Build history of the part. All positions in model axes, mm. A direction names the side the tool comes from. Round coordinates to 2 decimals unless told otherwise and drop trailing zeros. Loops run counter-clockwise (first coordinate to the right, second up) from the corner with the lowest first, then second, coordinate; pieces in that order, holes last.
Autodesk Inventor part; units mm, degrees
ref_plane "YZ Plane" through (0, 0, 0) normal (1, 0, 0) x (0, 1, 0)
ref_plane "XZ Plane" through (0, 0, 0) normal (0, 1, 0) x (-1, 0, 0)
ref_plane "XY Plane" through (0, 0, 0) normal (0, 0, 1) x (1, 0, 0)
sketch "Sketch1" plane through (0, 0, 0) normal (0, 1, 0) x (-1, 0, 0)
  line L0 (20.25, -20.25) -> (-20.25, -20.25)
  line L1 (-20.25, -20.25) -> (-20.25, 20.25)
  line L2 (-20.25, 20.25) -> (20.25, 20.25)
  line L3 (20.25, 20.25) -> (20.25, -20.25)
  line L4 (23.25, 23.25) -> (-23.25, 23.25)
  line L5 (-23.25, 23.25) -> (-23.25, -23.25)
  line L6 (-23.25, -23.25) -> (23.25, -23.25)
  line L7 (23.25, -23.25) -> (23.25, 23.25)
  point P0 (0, 0)
  point P1 (20.25, 0)
  point P2 (0, -20.25)
  point P3 (23.25, 0)
  point P4 (0, -23.25)
  dimension "d0" = 40.5
  dimension "d1" = 40.5
  dimension "d2" = 46.5
  dimension "d3" = 46.5
extrude "Extrusion1" add sketch "Sketch1" along normal blind 10
fillet "Fillet1" radius 3 8 edges at (-23.25, 5, 23.25) (23.25, 5, 23.25) (23.25, 5, -23.25) (-23.25, 5, -23.25) (-20.25, 5, -20.25) (-20.25, 5, 20.25) (20.25, 5, 20.25) (20.25, 5, -20.25)
ref_plane "Arbeitsebene3" through (-17.25, 0, -20.25) normal (1, 0, 0) x (0, 1, 0)
sketch "Skizze10" plane through (0, 10, 0) normal (0, 1, 0) x (1, 0, 0)
  line L0 (20.25, 23.25) -> (-20.25, 23.25)
  arc A0 (-20.25, 23.25) -> (-23.25, 20.25) centre (-20.25, 20.25) ccw
  line L1 (-23.25, 20.25) -> (-23.25, -20.25)
  arc A1 (-23.25, -20.25) -> (-20.25, -23.25) centre (-20.25, -20.25) ccw
  line L2 (-20.25, -23.25) -> (20.25, -23.25)
  arc A2 (20.25, -23.25) -> (23.25, -20.25) centre (20.25, -20.25) ccw
  line L3 (23.25, -20.25) -> (23.25, 20.25)
  arc A3 (23.25, 20.25) -> (20.25, 23.25) centre (20.25, 20.25) ccw
  line L4 (-20.25, 23.25) -> (20.25, 23.25)
  line L5 (23.25, 20.25) -> (23.25, -20.25)
  line L6 (20.25, -23.25) -> (-20.25, -23.25)
  line L7 (-23.25, -20.25) -> (-23.25, 20.25)
  arc A4 (-20.25, 23.25) -> (-23.25, 20.25) centre (-20.25, 20.25) ccw
  arc A5 (23.25, 20.25) -> (20.25, 23.25) centre (20.25, 20.25) ccw
  arc A6 (20.25, -23.25) -> (23.25, -20.25) centre (20.25, -20.25) ccw
  arc A7 (-23.25, -20.25) -> (-20.25, -23.25) centre (-20.25, -20.25) ccw
  line L8 (-20.25, -23.25) -> (20.25, -23.25)
  point P0 (0, 0)
extrude "Extrusion6" add sketch "Skizze10" along normal blind 2
sketch "Skizze9" plane through (-17.25, 0, -20.25) normal (1, 0, 0) x (0, 1, 0)
  line L0 (12, 0) -> (0, 0) construction
  line L1 (6.2, 0) -> (6.2, 0.8787) construction
  line L2 (3.3, 0) -> (1.3, 0)
  line L3 (10, 3) -> (10, 37.5)
  line L4 (10, 20.25) -> (0, 20.25)
  line L5 (10, 40.5) -> (0, 40.5) construction
  ellipse E0 centre (2.3, 0) end of major axis (1.3, 0) minor radius 0.5
  line L6 (3.3, 0) -> (1.3, 0)
  line L7 (10, 40.5) -> (0, 40.5) construction
  line L8 (3.3, 40.5) -> (1.3, 40.5)
  ellipse E1 centre (2.3, 40.5) end of major axis (1.3, 40.5) minor radius 0.5
  point P0 (4.6, 0)
  point P1 (10, 0)
  point P2 (6.2, 3)
  point P3 (6.2, 15.294)
  point P4 (2.3, 0.5)
  dimension "d51" = 1.6
  dimension "d52" = 2.3
  dimension "d53" = 1
  dimension "d64" = 0.5
chamfer "Fasen1" distance 2 angle 45 8 edges at (-23.25, 12, 0) (-22.3713, 12, 22.3713) (0, 12, 23.25) (22.3713, 12, 22.3713) (23.25, 12, 0) (22.3713, 12, -22.3713) (0, 12, -23.25) (-22.3713, 12, -22.3713)
extrude "Extrusion7" add sketch "Skizze9" along normal blind 37.5 and the other way blind 5 contours L2 E0 | E1 L8 picked at (2.2882, 0.1666) picked at (2.3118, 40.3334)
properties part number "IMU_mount_cover"
(1) Probe line 1 (Z direction, x = -4, y = 8); line 2 (X direction, y = 8, z = -17.5); line 3 (Y direction, x = 8.5, z = -5). List the from-to ranges inside material, lowest first.
Responses:
line 1: z = -23.25 to -20.25, 20.25 to 23.25
line 2: x = -23.25 to -20.24, 20.24 to 23.25
line 3: y = 10 to 12
(2) Which spindle directions (+Z, -Z, +X, -X, +Y, -Y) get a long thin tool onto all of the face, cutting with end or side? Do faces 1 (the face through (0, 1, -20.25)), 2 (the face through (-22.35, 4.93, 22.39)), 3 (the face through (19.35, 5.07, 19.39)). Say none if no direction does.
Responses:
face 1: -Y
face 2: +Z, -X, +Y, -Y
face 3: none
(3) Slice it at B-B on z = -16. List the corners of the cut face in (x, y).
Responses:
outline: (-23.25, 0) - (-20.25, 0) - (-20.25, 10) - (20.25, 10) - (20.25, 0) - (23.25, 0) - (23.25, 10) - (21.25, 12) - (-21.25, 12) - (-23.25, 10) - close
(4) Slice it at A-A on y = 6.75. List the corners of the cut face in (x, z).
Responses:
outline: (-23.25, -20.25) arc R3 ccw to (-20.25, -23.25) - (20.25, -23.25) arc R3 ccw to (23.25, -20.25) - (23.25, 20.25) arc R3 ccw to (20.25, 23.25) - (-20.25, 23.25) arc R3 ccw to (-23.25, 20.25) - close; hole (-20.25, -17.25) arc R3 ccw to (-17.25, -20.25) - (17.25, -20.25) arc R3 ccw to (20.25, -17.25) - (20.25, 17.25) arc R3 ccw to (17.25, 20.25) - (-17.25, 20.25) arc R3 ccw to (-20.25, 17.25) - close
(5) Pull direction X, two halves, no side cores. Call faces 4 (the face through (20.25, 5, 0)), 5 (the face through (-22.39, 4.93, -22.35)), 6 (the face through (23.25, 5, 0)), 7 (the face through (19.39, 5.07, -19.35)): +X half, -X half, draft (parallel to the pull), parting line (faces both ways), or undercut.
Responses:
face 4: undercut
face 5: -X half
face 6: +X half
face 7: undercut
(6) Pin check, flat tips, straight feed: P1, Ø20, axis at x = 3, z = -7.5, coming from the -Y side; P2, Ø4, axis at x = -14.5, z = -18, coming from the -Y side. Stop position of each tip, or through.
Responses:
P1: stops at y = 10
P2: stops at y = 1.43
